Verification items for the finished model (mm, model axes). Give positions to 0.01 mm unless a question says otherwise; leave off trailing zeros. Order: outer loops, then holes, each group sorted by start corner. A loop starts at its lowest first (then second) coordinate and runs counter-clockwise, first axis right, second up. Notation, with made-up numbers: M -5,-35.5 L 18,-35.5 A30 ccw 18,-4.5 Z; hole C 29.25,-11 d10. An arc over 180 degrees is marked long. Answer as a JSON object with one key per item and string values.
```python
from build123d import *


with BuildPart() as f3:
    # F0 (on Top) → F3 section 0
    with BuildSketch(Plane.XY):
        Polygon((65, 28.6817904562), (20, 40.2744300663), (-20, 40.2744300663), (-65, 28.6817904562), (-65, -17.7070442587), (-58.7742775679, -66.0424605012), (-30, -124.7455254197), (30, -124.7455254197), (58.7742775679, -66.0424605012), (65, -17.7070442587), align=None)
    # F2 (on offset) → F3 section 1
    with BuildSketch(Plane.XY.offset(10)):
        Polygon((58.7742775679, -71.0424605012), (65, -22.7070442587), (65, 23.6817904562), (20, 35.2744300663), (-20, 35.2744300663), (-65, 23.6817904562), (-65, -22.7070442587), (-58.7742775679, -71.0424605012), (-30, -129.7455254197), (30, -129.7455254197), align=None)
    loft()

    # F33: F3 across plane


with BuildPart() as f3_1:
    add(f3.part)
    add(f3.part.mirror(Plane.YZ))


solid = f3_1.part
```
Q1. Material ranges on L1, parallel to X at y = -84.5, z = 4.75; L2, parallel to Y at x = 3.5, z = 5.75; L3, parallel to Y at x = 6, z = 4.5, recorded low to high.
Resolved:
{"L1": "x = -50.89 to 50.89", "L2": "y = -127.62 to 37.4", "L3": "y = -127 to 38.02"}
Q2. Section check A-A on x = 13. Record the cut outline in (y, z).
Resolved:
{"outline": "M -129.75,10 L -124.75,0 L 40.27,0 L 35.27,10 Z"}
Q3. Gauge pin test, flat ends, axial feed: pin 1 Ø3 at (x, y) = (31.5, -58.5) entering from -Z; pin 2 Ø2 at (x, z) = (34.5, 5) entering from +Y. Record the tip position at first contact, or that the pin passes through.
Resolved:
{"pin 1": "stops at z = 0", "pin 2": "stops at y = 34.6"}
